```python
from build123d import *

# Parameters (mm, degrees)
ESQUISSE1_W             = 36
ESQUISSE1_H             = 36
ESQUISSE1_R             = 1.1
ESQUISSE1_R_2           = 4
ESQUISSE1_R_3           = 1.6
BOSS_EXTRU_1_DEPTH      = 3
ESQUISSE2_R             = 3
BOSS_EXTRU_2_DEPTH      = 2
ESQUISSE3_R             = 1.6
ENL_V_MAT_EXTRU_1_DEPTH = 26.942243542
CONG_1_R                = 2


with BuildPart() as part:
    # Esquisse1 → Boss.-Extru.1 (new body)
    with BuildSketch(Plane.XY):
        Rectangle(ESQUISSE1_W, ESQUISSE1_H)
        with Locations((-4.242640687, 4.242640687)):
            Circle(ESQUISSE1_R, mode=Mode.SUBTRACT)
        with Locations((4.242640687, 4.242640687)):
            Circle(ESQUISSE1_R, mode=Mode.SUBTRACT)
        with Locations((4.242640687, -4.242640687)):
            Circle(ESQUISSE1_R, mode=Mode.SUBTRACT)
        with Locations((-4.242640687, -4.242640687)):
            Circle(ESQUISSE1_R, mode=Mode.SUBTRACT)
        Circle(ESQUISSE1_R_2, mode=Mode.SUBTRACT)
        with Locations((-15, 15)):
            Circle(ESQUISSE1_R_3, mode=Mode.SUBTRACT)
        with Locations(Location((15, 15, 0), (0, 0, 180))):
            Circle(ESQUISSE1_R_3, mode=Mode.SUBTRACT)
        with Locations((15, -15)):
            Circle(ESQUISSE1_R_3, mode=Mode.SUBTRACT)
        with Locations(Location((-15, -15, 0), (0, 0, 180))):
            Circle(ESQUISSE1_R_3, mode=Mode.SUBTRACT)
    extrude(amount=BOSS_EXTRU_1_DEPTH)

    # Esquisse2 → Boss.-Extru.2 (add)
    with BuildSketch(Plane.XY.offset(3)):
        with Locations((-8, 8)):
            Circle(ESQUISSE2_R)
        with Locations((8, 8)):
            Circle(ESQUISSE2_R)
        with Locations((8, -8)):
            Circle(ESQUISSE2_R)
        with Locations((-8, -8)):
            Circle(ESQUISSE2_R)
    extrude(amount=BOSS_EXTRU_2_DEPTH)

    # Esquisse3 → Enlèv. mat.-Extru.1 (cut, through all)
    with BuildSketch(Plane.XY.offset(5)):
        with Locations((-8, 8)):
            Circle(ESQUISSE3_R)
        with Locations(Location((8, 8, 0), (0, 0, 180))):
            Circle(ESQUISSE3_R)
        with Locations((8, -8)):
            Circle(ESQUISSE3_R)
        with Locations(Location((-8, -8, 0), (0, 0, 180))):
            Circle(ESQUISSE3_R)
    extrude(amount=-ENL_V_MAT_EXTRU_1_DEPTH, mode=Mode.SUBTRACT)

    # Congé1
    cong_1_edges = [part.edges().sort_by_distance(p)[0] for p in [
        (-18, 18, 1.5),
        (18, 18, 1.5),
        (18, -18, 1.5),
        (-18, -18, 1.5),
    ]]
    fillet(cong_1_edges, radius=CONG_1_R)


solid = part.part
```
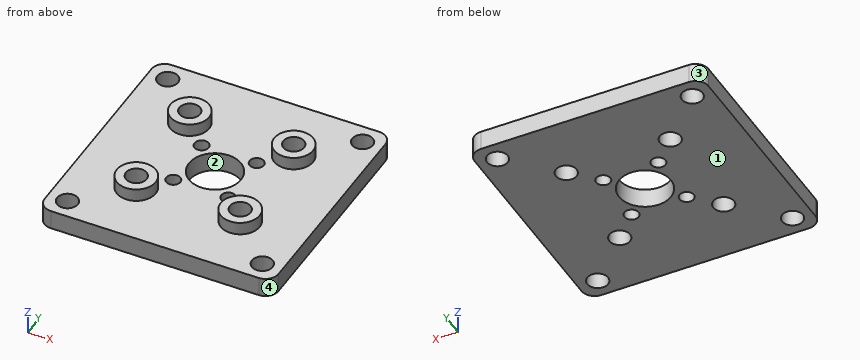
Can you work these out from the model? Positions are in its coordinate system, mm. Face numbers are marked on the shaded views. Coordinates: 2 decimals unless noted, no trailing zeros. Loops run counter-clockwise (first coordinate to the right, second up) from the corner with the lowest first, then second, coordinate; pieces in that order, holes last.
1) Thinking about a two-plate mould opening in X: for the marked faces 1, 2, 3 and 4, which applies, pulls with the +X half, pulls with the -X half, needs draft (parallel to the pull), parting line crosses it, or undercut?
2) For pin 1 (1.9 mm diameter, centred on x = 15, y = 15, fed in from -Z); pin 2 (5 mm diameter, centred on x = -1.5, y = -0.5, fed in from +Z), each with a flat end and sliding along its axis, tell me the tip position at first contact or that it passes through.
3) I need wall thicknesses on probe 1 along Y at (x, z) = (-8, 1.4); probe 2 along Y at (x, z) = (15, 2.35); probe 3 along X at (y, z) = (9, 0.85). Which ranges of each line are inside material? Lowest first, please.
4) Imagine slicing it at B-B on x = 8. List the corners of the cut face in (y, z) for me, plus the area to 3 significant figures.
5) Imagine slicing it at A-A on y = 15. List the corners of the cut face in (x, z) for me.
Completed:
1. face 1: needs draft
1. face 2: undercut
1. face 3: pulls with the -X half
1. face 4: pulls with the +X half
2. pin 1: passes through
2. pin 2: stops at z = 3
3. probe 1: y = -18 to -9.6, -6.4 to 6.4, 9.6 to 18
3. probe 2: y = -18 to -16.6, -13.4 to 13.4, 16.6 to 18
3. probe 3: x = -18 to -9.25, -6.75 to 6.75, 9.25 to 18
4. outline: (-18, 0) - (-9.6, 0) - (-9.6, 5) - (-11, 5) - (-11, 3) - (-18, 3) - close; (-6.4, 0) - (6.4, 0) - (6.4, 5) - (5, 5) - (5, 3) - (-5, 3) - (-5, 5) - (-6.4, 5) - close; (9.6, 0) - (18, 0) - (18, 3) - (11, 3) - (11, 5) - (9.6, 5) - close
4. area: 100 mm2
5. outline: (-18, 0) - (-16.6, 0) - (-16.6, 3) - (-18, 3) - close; (-13.4, 0) - (13.4, 0) - (13.4, 3) - (-13.4, 3) - close; (16.6, 0) - (18, 0) - (18, 3) - (16.6, 3) - close
